Input: part model. Units: mm. Frame: model coordinates. A direction names the side the tool comes from. Coordinates: 2 decimals unless noted, no trailing zeros. Loops run counter-clockwise (first coordinate to the right, second up) from the corner with the lowest first, then second, coordinate; pieces in that order, holes last.
Item 1: Reachability of faces 5 (the flat face through (-9, 41.75, 11)), 6 (the cylindrical face through (29.07, 47, 0.99)), 7 (the cylindrical face through (36.242, 38.463, 17.535)), 8 (the cylindrical face through (-18.96, -41.51, 8.2)) from +Z, -Z, +X, -X, +Y, -Y: full face, straight path, thin tool, end or side. Return the list, or none.
Item 2: Section B-B on y = -23. Return loops of the section in (x, z), and give its area (3 significant figures).
Item 3: Pull-direction query (X, two-part tool) for faces 1 (the flat face through (-40.5, 0, 11)), 2 (the cylindrical face through (-41, 41.07, 10.87)), 3 (the cylindrical face through (36.242, -34.537, 17.535)), 4 (the flat face through (-1, 42.5, 15)); classes: released by +X, released by -X, zero draft, split by the parting line, or undercut.
Item 4: Section D-D on y = -9.5. Return loops of the section in (x, z).
Item 5: Section A-A on x = -14. Return loops of the section in (y, z).
Item 6: Ray query, line 1 along Y through (x, z) = (36.5, 16.4); line 2 along Y through (x, z) = (29, 13.25); line 3 along X through (y, z) = (-37, 4.5). Return the intervals inside material, ascending.
Item 7: Contact query for flat-ended pins moving along their axis: P1, Ø1, axis at x = -12.5, z = 0.5, coming from the -Y side; P2, Ø2.5, axis at x = 37.5, z = 13, coming from the -Y side; P3, Ø1.9, axis at x = 10, z = 8.5, coming from the +Y side. Output: stop coordinate, or through.
Item 8: Section C-C on x = -4. Return loops of the section in (y, z).
```python
from build123d import *

# Parameters (mm, degrees)
PAD_DEPTH       = 20
POCKET_DEPTH    = 18
SKETCH003_R     = 1.6891
POCKET001_DEPTH = 10
SKETCH005_R     = 1.98
POCKET002_DEPTH = 5
SKETCH006_R     = 3
PAD001_DEPTH    = 8
SKETCH007_R     = 1.15
POCKET003_DEPTH = 7
SKETCH008_R     = 6.25
POCKET004_DEPTH = 5
POCKET008_DEPTH = 5
SKETCH013_R     = 4.40055
POCKET009_DEPTH = 0.75
SKETCH014_R     = 3.175
PAD002_DEPTH    = 2
SKETCH015_W     = 23.5
SKETCH015_H     = 6.3
POCKET010_DEPTH = 0.75
SKETCH016_W     = 16
SKETCH016_H     = 7.5
POCKET011_DEPTH = 5
SKETCH017_R     = 0.75
POCKET012_DEPTH = 5


with BuildPart() as part:
    # Sketch → Pad (new body)
    with BuildSketch(Plane.XY):
        with BuildLine():
            Line((-37.5, 42.5), (37.5, 42.5))
            ThreePointArc((42.5, 37.5), (41.035534, 41.035534), (37.5, 42.5))
            Line((42.5, 37.5), (42.5, -37.5))
            ThreePointArc((37.5, -42.5), (41.035534, -41.035534), (42.5, -37.5))
            Line((37.5, -42.5), (-37.5, -42.5))
            ThreePointArc((-42.5, -37.5), (-41.035534, -41.035534), (-37.5, -42.5))
            Line((-42.5, -37.5), (-42.5, 37.5))
            ThreePointArc((-37.5, 42.5), (-41.035534, 41.035534), (-42.5, 37.5))
        make_face()
    extrude(amount=PAD_DEPTH)

    # Sketch002 (on Face10 of Pad) → Pocket (cut)
    with BuildSketch(Plane.XY.offset(20)):
        with BuildLine():
            Line((-40.5, 30.5), (-40.5, -30.5))
            Line((-40.5, -30.5), (-35.5, -30.5))
            ThreePointArc((-30.5, -35.5), (-31.964466, -31.964466), (-35.5, -30.5))
            Line((-30.5, -35.5), (-30.5, -40.5))
            Line((-30.5, -40.5), (30.5, -40.5))
            Line((30.5, -40.5), (30.5, -35.5))
            ThreePointArc((35.5, -30.5), (31.964466, -31.964466), (30.5, -35.5))
            Line((35.5, -30.5), (40.5, -30.5))
            Line((40.5, -30.5), (40.5, 30.5))
            Line((40.5, 30.5), (35.5, 30.5))
            ThreePointArc((30.5, 35.5), (31.964466, 31.964466), (35.5, 30.5))
            Line((30.5, 35.5), (30.5, 40.5))
            Line((30.5, 40.5), (-30.5, 40.5))
            Line((-30.5, 40.5), (-30.5, 35.5))
            ThreePointArc((-35.5, 30.5), (-31.964466, 31.964466), (-30.5, 35.5))
            Line((-35.5, 30.5), (-40.5, 30.5))
        make_face()
    extrude(amount=-POCKET_DEPTH, mode=Mode.SUBTRACT)

    # Sketch003 (on Face5 of Pocket) → Pocket001 (cut)
    with BuildSketch(Plane.XY.offset(20)):
        with Locations((-36.5, 36.5)):
            Circle(SKETCH003_R)
        with Locations((36.5, 36.5)):
            Circle(SKETCH003_R)
        with Locations((36.5, -36.5)):
            Circle(SKETCH003_R)
        with Locations((-36.5, -36.5)):
            Circle(SKETCH003_R)
    extrude(amount=-POCKET001_DEPTH, mode=Mode.SUBTRACT)

    # Sketch005 (on Face5 of Pocket001) → Pocket002 (cut)
    with BuildSketch(Plane.XY.offset(20)):
        with Locations((-36.5, 36.5)):
            Circle(SKETCH005_R)
        with Locations((-36.5, -36.5)):
            Circle(SKETCH005_R)
        with Locations((36.5, -36.5)):
            Circle(SKETCH005_R)
        with Locations((36.5, 36.5)):
            Circle(SKETCH005_R)
    extrude(amount=-POCKET002_DEPTH, mode=Mode.SUBTRACT)

    # Sketch006 (on Face32 of Pocket002) → Pad001 (join)
    with BuildSketch(Plane.XY.offset(2)):
        with Locations((-33, 10)):
            Circle(SKETCH006_R)
        with Locations((33, 10)):
            Circle(SKETCH006_R)
        with Locations((-33, -23)):
            Circle(SKETCH006_R)
        with Locations((33, -23)):
            Circle(SKETCH006_R)
    extrude(amount=PAD001_DEPTH)

    # Sketch007 (on Face47 of Pad001) → Pocket003 (cut)
    with BuildSketch(Plane.XY.offset(10)):
        with Locations((33, 10)):
            Circle(SKETCH007_R)
        with Locations((33, -23)):
            Circle(SKETCH007_R)
        with Locations((-33, 10)):
            Circle(SKETCH007_R)
        with Locations((-33, -23)):
            Circle(SKETCH007_R)
    extrude(amount=-POCKET003_DEPTH, mode=Mode.SUBTRACT)

    # Sketch008 (on Face6 of Pocket003) → Pocket004 (cut)
    with BuildSketch(Plane.XZ.offset(42.5)):
        with Locations((-14, 12)):
            Circle(SKETCH008_R)
        with Locations((14, 12)):
            Circle(SKETCH008_R)
    extrude(amount=-POCKET004_DEPTH, mode=Mode.SUBTRACT)

    # Sketch012 → Pocket008 (cut)
    with BuildSketch(Plane(origin=(-42.5, 0, 0), x_dir=(0, -1, 0), z_dir=(-1, 0, 0))):
        with BuildLine():
            ThreePointArc((-19.4346, 11.692486), (-25.0734, 10), (-19.4346, 8.307514))
            Line((-19.4346, 11.692486), (-19.4346, 8.307514))
        make_face()
    extrude(amount=-POCKET008_DEPTH, mode=Mode.SUBTRACT)

    # Sketch013 (on Face1 of Pocket008) → Pocket009 (cut)
    with BuildSketch(Plane(origin=(-42.5, 0, 0), x_dir=(0, -1, 0), z_dir=(-1, 0, 0))):
        with Locations((-22, 10)):
            Circle(SKETCH013_R)
    extrude(amount=-POCKET009_DEPTH, mode=Mode.SUBTRACT)

    # Sketch014 (on Face3 of Pocket009) → Pad002 (join)
    with BuildSketch(Plane(origin=(0, 0, 0), x_dir=(1, 0, 0), z_dir=(0, 0, -1))):
        with BuildLine():
            ThreePointArc((-30.5, 50.5), (-36.5, 56.5), (-42.5, 50.5))
            Line((-42.5, 50.5), (-42.5, -50.5))
            ThreePointArc((-42.5, -50.5), (-36.5, -56.5), (-30.5, -50.5))
            ThreePointArc((-25.5, -45.5), (-29.035534, -46.964466), (-30.5, -50.5))
            Line((-25.5, -45.5), (25.5, -45.5))
            ThreePointArc((30.5, -50.5), (29.035534, -46.964466), (25.5, -45.5))
            ThreePointArc((30.5, -50.5), (36.5, -56.5), (42.5, -50.5))
            Line((42.5, -50.5), (42.5, 50.5))
            ThreePointArc((42.5, 50.5), (36.5, 56.5), (30.5, 50.5))
            ThreePointArc((25.5, 45.5), (29.035534, 46.964466), (30.5, 50.5))
            Line((-25.5, 45.5), (25.5, 45.5))
            ThreePointArc((-30.5, 50.5), (-29.035534, 46.964466), (-25.5, 45.5))
        make_face()
        with Locations((-36.5, -50.5)):
            Circle(SKETCH014_R, mode=Mode.SUBTRACT)
        with Locations((36.5, -50.5)):
            Circle(SKETCH014_R, mode=Mode.SUBTRACT)
        with Locations((36.5, 50.5)):
            Circle(SKETCH014_R, mode=Mode.SUBTRACT)
        with Locations((-36.5, 50.5)):
            Circle(SKETCH014_R, mode=Mode.SUBTRACT)
    extrude(amount=-PAD002_DEPTH)

    # Sketch015 → Pocket010 (cut)
    with BuildSketch(Plane(origin=(0, 42.5, 0), x_dir=(-1, 0, 0), z_dir=(0, 1, 0))):
        with Locations((0, 10)):
            Rectangle(SKETCH015_W, SKETCH015_H)
    extrude(amount=-POCKET010_DEPTH, mode=Mode.SUBTRACT)

    # Sketch016 (on Face32 of Pocket010) → Pocket011 (cut)
    with BuildSketch(Plane(origin=(0, 42.5, 0), x_dir=(-1, 0, 0), z_dir=(0, 1, 0))):
        with Locations((0, 10)):
            Rectangle(SKETCH016_W, SKETCH016_H)
    extrude(amount=-POCKET011_DEPTH, mode=Mode.SUBTRACT)

    # Sketch017 (on Face77 of Pocket011) → Pocket012 (cut)
    with BuildSketch(Plane(origin=(0, 41.75, 0), x_dir=(-1, 0, 0), z_dir=(0, 1, 0))):
        with Locations((-9.875, 10)):
            Circle(SKETCH017_R)
        with Locations((9.875, 10)):
            Circle(SKETCH017_R)
    extrude(amount=-POCKET012_DEPTH, mode=Mode.SUBTRACT)


solid = part.part
```
Results found:
1. face 5: +Y
1. face 6: +Z, -Z, +Y
1. face 7: +Z
1. face 8: -Y
2. outline: (-42.5, 0) - (42.5, 0) - (42.5, 20) - (40.5, 20) - (40.5, 2) - (36, 2) - (36, 10) - (34.15, 10) - (34.15, 3) - (31.85, 3) - (31.85, 10) - (30, 10) - (30, 2) - (-30, 2) - (-30, 10) - (-31.85, 10) - (-31.85, 3) - (-34.15, 3) - (-34.15, 10) - (-36, 10) - (-36, 2) - (-40.5, 2) - (-40.5, 20) - (-42.5, 20) - close
2. area: 306 mm2
3. face 1: undercut
3. face 2: released by -X
3. face 3: undercut
3. face 4: zero draft
4. outline: (-42.5, 0) - (42.5, 0) - (42.5, 20) - (40.5, 20) - (40.5, 2) - (-40.5, 2) - (-40.5, 20) - (-42.5, 20) - close
5. outline: (-45.5, 0) - (45.5, 0) - (45.5, 2) - (42.5, 2) - (42.5, 20) - (40.5, 20) - (40.5, 2) - (-40.5, 2) - (-40.5, 5.75) - (-42.5, 5.75) - (-42.5, 2) - (-45.5, 2) - close; (-42.5, 18.25) - (-40.5, 18.25) - (-40.5, 20) - (-42.5, 20) - close
6. line 1: y = -42.5 to -38.48, -34.52 to -30.5, 30.5 to 34.52, 38.48 to 42.5
6. line 2: y = -42.5 to -40.5, 40.5 to 42.5
6. line 3: x = -42.5 to -30.5, 30.5 to 42.5
7. P1: stops at y = -45.5
7. P2: stops at y = -42.5
7. P3: stops at y = 41.75
8. outline: (-45.5, 0) - (45.5, 0) - (45.5, 2) - (42.5, 2) - (42.5, 6.25) - (40.5, 6.25) - (40.5, 2) - (-40.5, 2) - (-40.5, 20) - (-42.5, 20) - (-42.5, 2) - (-45.5, 2) - close; (40.5, 13.75) - (42.5, 13.75) - (42.5, 20) - (40.5, 20) - close
